Could you check a few things on this model? Use its own coordinates, in mm. Face numbers are marked on the shaded views. A direction names the side the tool comes from. Round coordinates to 2 decimals unless told otherwise and drop trailing zeros. Loops run counter-clockwise (first coordinate to the right, second up) from the corner with the lowest first, then second, coordinate; pieces in that order, holes last. Notation, with made-up numbers: (-27, -30) - (19, -30) arc R8 ccw to (19, -17) - close; hole circle Ø3 at (-27, 72.5). An arc over 180 degrees is marked (long way). Use one line per item in the form item = value.
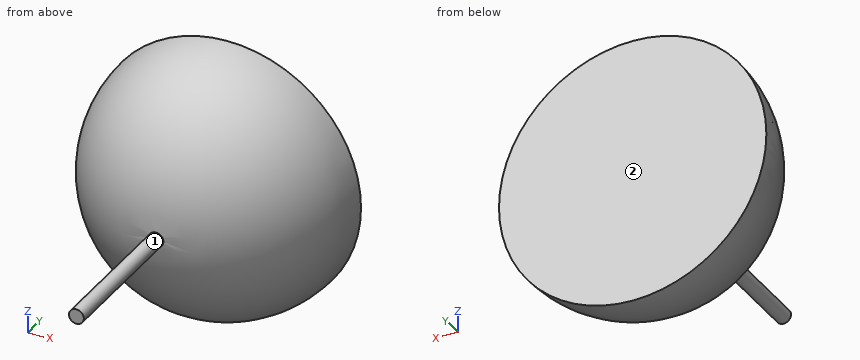
```python
from build123d import *

# Parameters (mm, degrees)
F2_R          = 1.27
F3_DEPTH      = 48.26
F3_DEPTH_BACK = 48.26
F4_R          = 26.181924
F5_DEPTH      = 48.261


with BuildPart() as f1:
    # F0 (on Front) → F1 (revolve)
    with BuildSketch(Plane.XZ):
        with BuildLine():
            Line((0, 22.86), (0, -22.86))
            ThreePointArc((0, -22.86), (22.86, 0), (0, 22.86))
        make_face()
    revolve(axis=Axis((0, 0, 0), (0, 0, -1)))

    # F2 (on Front) → F3 (join, two sides)
    with BuildSketch(Plane.XZ) as f3_sk:
        Circle(F2_R)
    extrude(amount=F3_DEPTH)
    extrude(f3_sk.sketch, amount=-F3_DEPTH_BACK)

    # F4 (on Front) → F5 (cut, through all)
    with BuildSketch(Plane.XZ):
        Circle(F4_R)
    extrude(amount=-F5_DEPTH, mode=Mode.SUBTRACT)


solid = f1.part
```
1. If we section it at B-B, the plane z = 0: Write out the boundary of the cut face in (x, y).
Solution:
outline = (-22.86, 0) arc R22.86 ccw to (-1.27, -22.82) - (-1.27, -48.26) - (1.27, -48.26) - (1.27, -22.82) arc R22.86 ccw to (22.86, 0) - close
2. For P1, Ø1.5, axis at x = -14, z = 11.5, coming from the -Y side; P2, Ø1, axis at y = -40.5, z = -3, coming from the -X side; P3, Ø6, axis at x = 5.5, z = -17.5, coming from the -Y side; P4, Ø4, axis at y = -8, z = -8.5, coming from the +X side, each with a flat end and sliding along its axis, tell me the tip position at first contact or that it passes through.
Solution:
P1 = -14.86
P2 = through
P3 = -16.95
P4 = 20.71
3. If we section it at A-A, the plane x = 0: Write out the boundary of the cut face in (y, z).
Solution:
outline = (-48.26, -1.27) - (-22.82, -1.27) arc R22.86 ccw to (0, -22.86) - (0, 22.86) arc R22.86 ccw to (-22.82, 1.27) - (-48.26, 1.27) - close
4. Please list where these lines run through material, in increasing order: line 1 along X through (y, z) = (-1.5, -13); line 2 along Z through (x, y) = (0, -42); line 3 along Y through (x, z) = (-17, 12).
Solution:
line_1 = -18.74 to 18.74
line_2 = -1.27 to 1.27
line_3 = -9.46 to 0
5. If we section it at C-C, the plane y = -34: Write out the boundary of the cut face in (x, z).
Solution:
outline = circle Ø2.54 at (0, 0)
6. If we section it at D-D, the plane y = -18.5: Write out the boundary of the cut face in (x, z).
Solution:
outline = circle Ø26.86 at (0, 0)
7. On a 3-axis mill with a long thin cutter (end or side, diameter ignored), from which of +Z, -Z, +X, -X, +Y, -Y can I reach the whole of each face in a straight line? I mean the marked faces 1 and 2. Say none if no direction works.
Solution:
face_1 = -Y
face_2 = +Z, -Z, +X, -X, +Y
